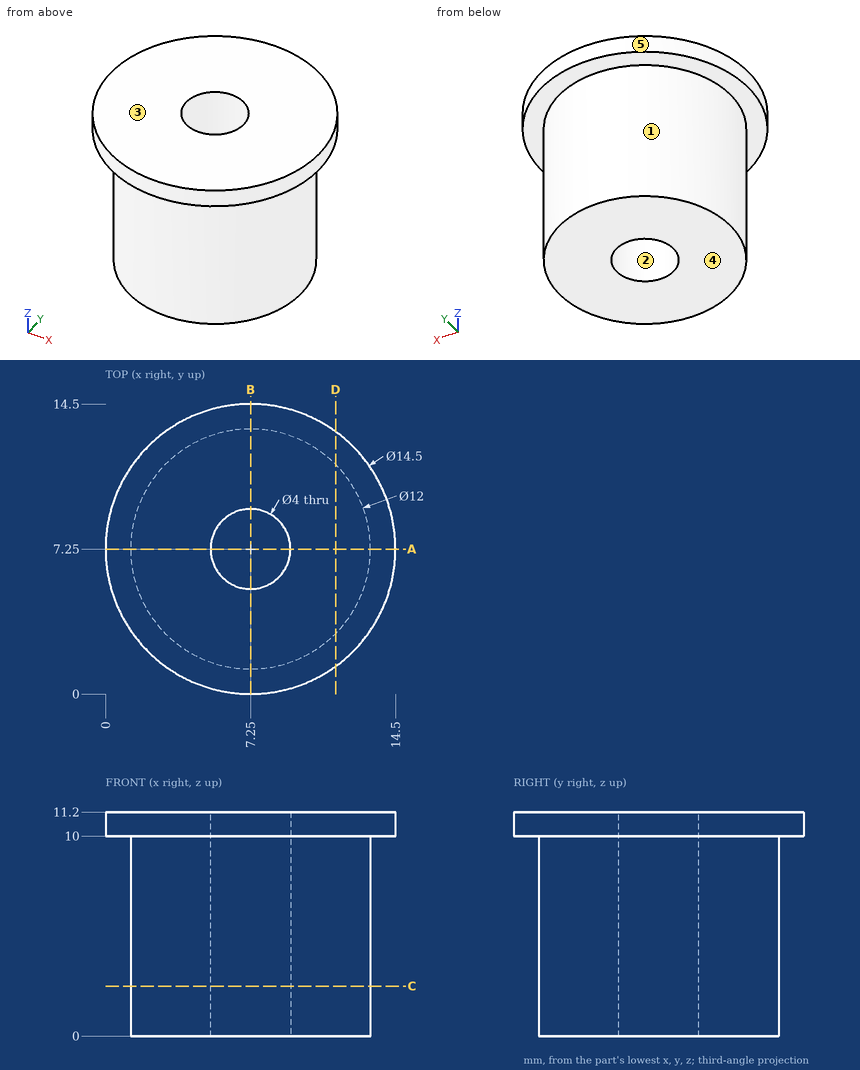
The drawing under review shows one solid part. Ordinate dimensions are in mm from its lowest x, y, z. A direction names the side the tool comes from. Coordinates: 2 decimals unless noted, no trailing zeros. Write each loop counter-clockwise with the first axis right and the second up, starting at its lowest first coordinate (ties: lowest second). Pieces come first, ordered by that corner, then holes. Notation, with made-up numbers: M 87.25,-26.75 L 137.25,-26.75 A14 ccw 137.25,-1.75 Z; hole C 79,-9 d11. An arc over 180 degrees is marked long. Answer as a JSON object with one key per item and string values.
Item 1: Add section D-D, the plane x = 11.5. Give the boundary of the cut face in (y, z).
Outcome:
{"outline": "M 1.38,10 L 3.01,10 L 3.01,0 L 11.49,0 L 11.49,10 L 13.12,10 L 13.12,11.2 L 1.38,11.2 Z"}
Item 2: Add section A-A, the plane y = 7.25. Give the boundary of the cut face in (x, z).
Outcome:
{"outline": "M 0,10 L 1.25,10 L 1.25,0 L 5.25,0 L 5.25,11.2 L 0,11.2 Z; M 9.25,0 L 13.25,0 L 13.25,10 L 14.5,10 L 14.5,11.2 L 9.25,11.2 Z"}
Item 3: Insertion check: pin 1 Ø4 at (y, z) = (10.5, 5) entering from -X; pin 2 Ø4 at (x, z) = (3, 9.5) entering from +Y; pin 3 Ø4 at (x, z) = (9, 2.5) entering from -Y. Each pin has a flat end and moves straight along its axis. Give the tip position at first contact, or say it passes through.
Outcome:
{"pin 1": "x = 1.38", "pin 2": "y = 14.12", "pin 3": "y = 1.25"}
Item 4: Machinability: for the marked faces 1 and 2, which of the approach directions +Z, -Z, +X, -X, +Y, -Y give a long, thin tool a straight path to every point of the face, cutting with its end or side? Answer none if there is none.
Outcome:
{"face 1": "-Z", "face 2": "+Z, -Z"}
Item 5: Draft analysis for pull direction Z (two halves, no side actions). For the marked faces 3, 4 and 5, state which applies: pulls with the +Z half, pulls with the -Z half, needs draft (parallel to the pull), parting line crosses it, or undercut.
Outcome:
{"face 3": "pulls with the +Z half", "face 4": "pulls with the -Z half", "face 5": "needs draft"}
Item 6: Add section C-C, the plane z = 2.5. Give the boundary of the cut face in (x, y), and give its area (3 significant figures).
Outcome:
{"outline": "C 7.25,7.25 d12; hole C 7.25,7.25 d4", "area": "101 mm²"}
Item 7: Wall thickness on probe 1 along Y at (x, z) = (7.25, 5.5); probe 2 along X at (y, z) = (9, 10.25); probe 3 along Z at (x, y) = (4.75, 13.75): over which ranges is each line inside the solid? List them lowest first.
Outcome:
{"probe 1": "1.25 to 5.25, 9.25 to 13.25", "probe 2": "0.21 to 6.28, 8.22 to 14.29", "probe 3": "10 to 11.2"}
